Read the model definition and answer for the solid it produces. Units are mm, in the model's axes. Face numbers are marked on the shaded views. A direction names the side the tool comes from. Coordinates: 2 decimals unless noted, no trailing zeros. Write each loop counter-clockwise with the first axis right and the second up, starting at its lowest first coordinate (ties: lowest second). Pieces come first, ordered by that corner, then holes.
(1) Which of the six approach directions +Z, -Z, +X, -X, +Y, -Y give full straight-line access (tool end or side, diameter ignored) to the marked faces 1 and 2?
(2) Section A-A on z = 0 is taken. Write down the section's boundary in (x, y).
(3) Section B-B on x = 0 is taken. Write down the section's boundary in (y, z), then the cut area to 3 significant figures.
(4) The mould has two halves that part along X. Classify the marked faces 3, 4 and 5: +X half, -X half, draft (parallel to the pull), parting line (faces both ways), or undercut.
(5) Find the intervals of material crossed by probe 1 along Z at (x, y) = (0, 37.75); probe 2 along X at (y, z) = (3, 0); probe 3 along Y at (x, z) = (-3.5, -16), in increasing order.
(6) Section D-D on y = 16 is taken. Write down the section's boundary in (x, z), then the cut area to 3 significant figures.
(7) Section C-C on z = 11 is taken. Write down the section's boundary in (x, y), then the cut area to 3 significant figures.
(8) Given pin 1 (3 mm diameter, centred on x = 2.5, y = -10, fed in from -Z); pin 2 (12 mm diameter, centred on x = -10.5, y = 12.5, fed in from -Z); pin 3 (1 mm diameter, centred on y = 28, z = -8.5, fed in from -X), each flat-ended and moving along its own axis, determine where each tip first touches the part or whether it passes through.
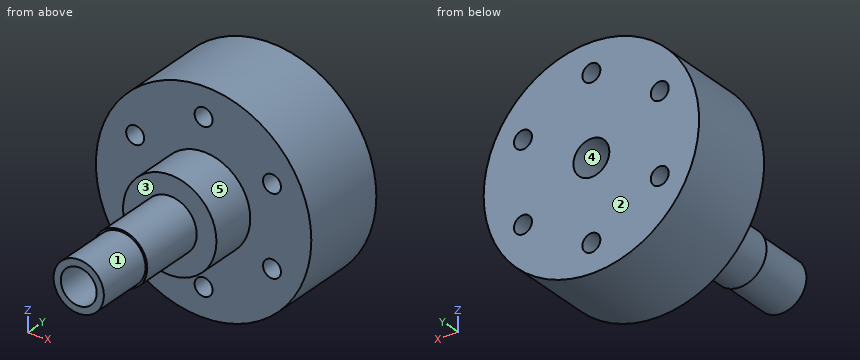
Autodesk Inventor part; units mm, degrees
ref_plane "YZ Plane" through (0, 0, 0) normal (1, 0, 0) x (0, 1, 0)
ref_plane "XZ Plane" through (0, 0, 0) normal (0, 1, 0) x (-1, 0, 0)
ref_plane "XY Plane" through (0, 0, 0) normal (0, 0, 1) x (1, 0, 0)
sketch "esq_rev" plane through (0, 0, 0) normal (0, 0, 1) x (1, 0, 0)
  line L0 (0, -40.1) -> (0, 62.1)
  line L1 (7.5, -9.5) -> (7.5, 9.5)
  line L2 (7.5, 9.5) -> (13, 9.5)
  line L3 (13, 9.5) -> (13, 22.5)
  line L4 (13, 22.5) -> (30, 22.5)
  line L5 (30, 22.5) -> (30, 47.5)
  line L6 (30, 47.5) -> (0, 47.5)
  line L7 (0, -25.5) -> (0, -0.0006)
  line L8 (-38.091, 0) -> (41.3485, 0)
  line L9 (-26.7425, 30) -> (-5.3911, 30)
  line L10 (-5.3911, 30) -> (28.4337, 30)
  line L11 (28.4337, 30) -> (7.0823, 30)
  line L12 (7.0823, 30) -> (-26.7425, 30)
  line L13 (-6.854, 30) -> (-23.5883, 30)
  line L14 (-23.5883, 30) -> (-14.3845, 30)
  line L15 (-4.5388, 30) -> (-6.854, 30)
  line L16 (-24.4454, 30) -> (5.2291, 30)
  line L17 (5.2291, 30) -> (2.6006, 30)
  line L18 (-13.9964, 30) -> (-24.4454, 30)
  line L19 (24.4454, 30) -> (-5.2291, 30)
  line L20 (-5.2291, 30) -> (-2.6006, 30)
  line L21 (13.9964, 30) -> (24.4454, 30)
  line L22 (4.5388, 30) -> (7.194, 30)
  line L23 (7.194, 30) -> (24.9396, 30)
  line L24 (24.9396, 30) -> (14.3845, 30)
  line L25 (-4.5388, 30) -> (-14.5, 30)
  line L26 (2.6006, 30) -> (-13.9964, 30)
  line L27 (13.9964, 30) -> (-2.6006, 30)
  line L28 (14.5, 30) -> (4.5388, 30)
  line L29 (-12.5, 30) -> (12.5, 30)
  line L30 (-12.5, -20) -> (12.5, -20)
  line L31 (7, -9.5) -> (7, -25.5)
  line L32 (7, -25.5) -> (0, -25.5)
  line L33 (7, -9.5) -> (7.5, -9.5)
  line L34 (0, -0.0006) -> (0, 47.5)
  point P0 (0, 0)
  dimension "d0" = 30
  dimension "d1" = 13
  dimension "d2" = 7.5
  dimension "d5" = 13
  dimension "d6" = 25
  dimension "d23" = 7
  dimension "d25" = 19
  dimension "d26" = 16
revolve "rev" add sketch "esq_rev" angle 360 about axis through (0, -25.5, 0) along (0, 1, 0)
sketch "esq_percage" plane through (0, 0, 0) normal (0, 1, 0) x (-1, 0, 0)
  line L0 (0, -7) -> (0, 7)
  line L1 (-7, 0) -> (7, 0)
  circle A0 centre (0, 0) radius 5
  dimension "d8" = 10
extrude "ext_percage" cut sketch "esq_percage" along normal through all both and the other way through all
sketch "Esq_trous" plane through (0, 0, 0) normal (0, 1, 0) x (-1, 0, 0)
  line L0 (0, -4.9) -> (0, 29.4)
  line L1 (-3.5, 0) -> (3.5, 0)
  circle A0 centre (0, 22) radius 2.5
  point P0 (0, 0)
  dimension "d11" = 5
  dimension "d12" = 22
extrude "ext_trous" cut sketch "Esq_trous" along normal through all
pattern_circular "Réseau circulaire1" count 6 over 360 about axis through (0, -10, 0) along (0, 1, 0) of "ext_trous"
thread "Filetage2"
properties part number "wheel_hub_spacer" material "Aluminium 6061"
Response:
1. face 1: -Y
1. face 2: +Z, -Z, +X, -X, +Y
2. outline: (-30, 22.5) - (-13, 22.5) - (-13, 9.5) - (-7.5, 9.5) - (-7.5, -9.5) - (-7, -9.5) - (-7, -25.5) - (-5, -25.5) - (-5, 47.5) - (-30, 47.5) - close; (5, -25.5) - (7, -25.5) - (7, -9.5) - (7.5, -9.5) - (7.5, 9.5) - (13, 9.5) - (13, 22.5) - (30, 22.5) - (30, 47.5) - (5, 47.5) - close
3. outline: (-25.5, -7) - (-9.5, -7) - (-9.5, -7.5) - (9.5, -7.5) - (9.5, -13) - (22.5, -13) - (22.5, -19.5) - (47.5, -19.5) - (47.5, -5) - (-25.5, -5) - close; (-25.5, 5) - (47.5, 5) - (47.5, 19.5) - (22.5, 19.5) - (22.5, 13) - (9.5, 13) - (9.5, 7.5) - (-9.5, 7.5) - (-9.5, 7) - (-25.5, 7) - close; (22.5, -30) - (47.5, -30) - (47.5, -24.5) - (22.5, -24.5) - close; (22.5, 24.5) - (47.5, 24.5) - (47.5, 30) - (22.5, 30) - close
3. area: 1,370 mm2
4. face 3: draft
4. face 4: undercut
4. face 5: parting line
5. probe 1: z = -30 to -24.5, -19.5 to -5, 5 to 19.5, 24.5 to 30
5. probe 2: x = -7.5 to -5, 5 to 7.5
5. probe 3: y = 22.5 to 47.5
6. outline: circle Ø26 at (0, 0); hole circle Ø10 at (0, 0)
6. area: 452 mm2
7. outline: (-27.91, 22.5) - (-21.55, 22.5) - (-21.55, 47.5) - (-27.91, 47.5) - close; (-16.55, 22.5) - (-6.93, 22.5) - (-6.93, 9.5) - (6.93, 9.5) - (6.93, 22.5) - (16.55, 22.5) - (16.55, 47.5) - (-16.55, 47.5) - close; (21.55, 22.5) - (27.91, 22.5) - (27.91, 47.5) - (21.55, 47.5) - close
7. area: 1,330 mm2
8. pin 1: stops at z = -7.42
8. pin 2: stops at z = -12.2
8. pin 3: stops at x = -28.91
